Can you work these out from the model? Positions are in its coordinate system, mm. A direction names the side the tool comes from. Give positions to 0.01 mm unless a question says otherwise; leave off trailing zeros. Write each loop counter-clockwise with the first axis right and the second up, starting at its lowest first coordinate (ties: lowest second). Pieces come first, ordered by that corner, then holes.
```python
from build123d import *

# Parameters (mm, degrees)
F1_DEPTH = 5.08
F2_R     = 2.6137383635
F2_R_2   = 1.27
F3_DEPTH = 1.016
F5_DEPTH = 0.4572
F6_R     = 1.5849178859
F6_R_2   = 1.5875
F7_DEPTH = 1.27
F9_DEPTH = 1.27


with BuildPart() as f1:
    # F0 (on Top) → F1 (new body)
    with BuildSketch(Plane.XY):
        with BuildLine():
            Line((-3.2727682094, 26.3807782884), (-6.4659603156, 19.0687214415))
            Line((-6.4659603156, 19.0687214415), (-30.863808468, 9.4360690564))
            ThreePointArc((-30.863808468, 9.4360690564), (-32.5086762666, 4.4664752799), (-27.325283736, 3.7351106293))
            Line((-27.325283736, 3.7351106293), (-6.8804663606, 11.2053323537))
            Line((-6.8804663606, 11.2053323537), (-6.8804663606, -7.0770513266))
            Line((-6.8804663606, -7.0770513266), (-21.0345704108, -28.5047926009))
            ThreePointArc((-21.0345704108, -28.5047926009), (-17.4572264743, -34.3414996844), (-11.008746922, -32.0433154702))
            Line((-11.008746922, -32.0433154702), (0, -13.9575190842))
            Line((0, -13.9575190842), (11.008746922, -32.0433154702))
            ThreePointArc((11.008746922, -32.0433154702), (17.4572264743, -34.3414996844), (21.0345704108, -28.5047926009))
            Line((21.0345704108, -28.5047926009), (6.8804663606, -7.0770513266))
            Line((6.8804663606, -7.0770513266), (6.8804663606, 11.2053323537))
            Line((6.8804663606, 11.2053323537), (27.325283736, 3.7351106293))
            ThreePointArc((27.325283736, 3.7351106293), (32.5086762666, 4.4664752799), (30.863808468, 9.4360690564))
            Line((30.863808468, 9.4360690564), (6.4659603156, 19.0687214415))
            Line((6.4659603156, 19.0687214415), (3.2727682094, 26.3807782884))
            ThreePointArc((3.2727682094, 26.3807782884), (0, 44.2043436195), (-3.2727682094, 26.3807782884))
        make_face()
    extrude(amount=F1_DEPTH)

    # F2 (on face) → F3 (join)
    with BuildSketch(Plane.XY.offset(5.08)):
        with Locations((-4.7121047974, 37.2473150492)):
            Circle(F2_R)
        with Locations((-4.7121047974, 37.2473150492)):
            Circle(F2_R_2, mode=Mode.SUBTRACT)
        with Locations((4.7121047974, 37.2473150492)):
            Circle(F2_R)
        with Locations((4.7121047974, 37.2473150492)):
            Circle(F2_R_2, mode=Mode.SUBTRACT)
        with BuildLine():
            Line((-3.2727682094, 30.2372745808), (-4.7121047974, 32.4515290558))
            ThreePointArc((-4.7121047974, 32.4515290558), (0.2937612268, 27.1153177061), (5.2996272509, 32.4515290558))
            Line((5.2996272509, 32.4515290558), (3.2727682094, 30.2372745808))
            Line((3.2727682094, 30.2372745808), (2.0341726185, 32.4515290558))
            Line((2.0341726185, 32.4515290558), (0, 30.2372745808))
            Line((0, 30.2372745808), (-1.5411652881, 32.4515290558))
            Line((-1.5411652881, 32.4515290558), (-3.2727682094, 30.2372745808))
        make_face()
        Polygon((-1.5411652881, 32.4515290558), (-4.7121047974, 32.4515290558), (-3.2727682094, 30.2372745808), align=None)
        Polygon((3.2727682094, 30.2372745808), (5.2996272509, 32.4515290558), (2.0341726185, 32.4515290558), align=None)
        Polygon((2.0341726185, 32.4515290558), (-1.5411652881, 32.4515290558), (0, 30.2372745808), align=None)
    extrude(amount=F3_DEPTH)

    # F4 (on face) → F5 (join)
    with BuildSketch(Plane.XY.offset(6.096)):
        with BuildLine():
            Line((-3.2727682094, 30.2372745808), (-4.7121047974, 32.4515290558))
            ThreePointArc((-4.7121047974, 32.4515290558), (-4.7203324358, 32.2729584869), (-4.7221920847, 32.0942081475))
            Line((-4.7221920847, 32.0942081475), (-3.4431374496, 30.126529098))
            Line((-3.4431374496, 30.126529098), (-3.2880254188, 29.8879070055))
            Line((-3.2880254188, 29.8879070055), (-3.1127018776, 30.1120986668))
            Line((-3.1127018776, 30.1120986668), (-1.5506819831, 32.1095020547))
            Line((-1.5506819831, 32.1095020547), (-0.1667791776, 30.121192946))
            Line((-0.1667791776, 30.121192946), (-0.0219153894, 29.9130612851))
            Line((-0.0219153894, 29.9130612851), (0.1496401921, 30.0998043917))
            Line((0.1496401921, 30.0998043917), (1.9938853204, 32.1073174174))
            Line((1.9938853204, 32.1073174174), (3.0954276532, 30.138074948))
            Line((3.0954276532, 30.138074948), (3.2517947624, 29.9134160007))
            Line((3.2517947624, 29.9134160007), (3.4226548069, 30.1000730943))
            Line((3.4226548069, 30.1000730943), (5.3097613024, 32.1616540513))
            ThreePointArc((5.3097613024, 32.1616540513), (5.306789943, 32.3066648182), (5.2996272509, 32.4515290558))
            Line((5.2996272509, 32.4515290558), (3.2727682094, 30.2372745808))
            Line((3.2727682094, 30.2372745808), (2.13859977, 32.2648431922))
            Line((2.13859977, 32.2648431922), (2.0341726185, 32.4515290558))
            Line((2.0341726185, 32.4515290558), (1.8894581688, 32.2940032811))
            Line((1.8894581688, 32.2940032811), (0, 30.2372745808))
            Line((0, 30.2372745808), (-1.4196918326, 32.2770032315))
            Line((-1.4196918326, 32.2770032315), (-1.5411652881, 32.4515290558))
            Line((-1.5411652881, 32.4515290558), (-1.6721554386, 32.2840278791))
            Line((-1.6721554386, 32.2840278791), (-3.2727682094, 30.2372745808))
        make_face()
    extrude(amount=F5_DEPTH)

    # F6 (on face) → F7 (join)
    with BuildSketch(Plane.XY.offset(5.08)):
        with Locations((0, 16.6316951297)):
            Circle(F6_R)
        with Locations((0, 10.2816951297)):
            Circle(F6_R_2)
        with Locations((0, 3.9316951297)):
            Circle(F6_R_2)
    extrude(amount=F7_DEPTH)

    # F8 (on face) → F9 (join)
    with BuildSketch(Plane.XY.offset(5.08)):
        with BuildLine():
            add(Edge.make_bspline(
                [(-7.0363054983, -4.8071318306), (-6.9812030221, -5.5234641768), (-6.9261005459, -6.239796523), (-6.8709980696, -6.9561288692)],
                knots=[0, 0, 0, 0, 2.1553456377, 2.1553456377, 2.1553456377, 2.1553456377], degree=3))
            add(Edge.make_bspline(
                [(-6.8709980696, -6.9561288692), (-5.6130342711, -8.3738225884), (-3.1848892901, -11.1102812153), (-0.243495057, -7.0612015798), (4.5821148023, -4.8991787577), (6.1734744422, -6.3428325856), (6.8495194428, -6.9561288692)],
                knots=[0, 0, 0, 0, 0.2686113424, 0.5184785791, 0.7954389812, 1, 1, 1, 1], degree=3))
            add(Edge.make_bspline(
                [(-7.0363054983, -4.8071318306), (-5.7248109737, -6.1236047459), (-3.2262965612, -8.6316034379), (-0.1133011688, -5.1968632917), (4.3194928458, -2.8270018136), (7.3601699927, -4.4068743135), (7.0165421861, -6.1223228754), (6.8495194428, -6.9561288692)],
                knots=[0, 0, 0, 0, 0.2276234559, 0.4336430496, 0.668963168, 0.8390971896, 1, 1, 1, 1], degree=3))
        make_face()
    extrude(amount=F9_DEPTH)


solid = f1.part
```
1) For pin 1 Ø2.5 at (x, y) = (5, 37.5) entering from +Z; pin 2 Ø3 at (y, z) = (29.5, 4) entering from +X; pin 3 Ø1 at (x, y) = (-5.5, 5.5) entering from +Z; pin 4 Ø5 at (x, y) = (-11, 7.5) entering from -Z, each with a flat end and sliding along its axis, tell me the tip position at first contact or that it passes through.
Values follow:
pin 1: stops at z = 6.1
pin 2: stops at x = 8.3
pin 3: stops at z = 5.08
pin 4: stops at z = 0
2) For faces 1 (the face through (0.2, 29.7, 6.096)), 2 (the face through (-13.86, -17.64, 2.5)), 3 (the face through (4, 32, 6.096)), which set-ups out of +Z, -Z, +X, -X, +Y, -Y let a thin tool reach every point of the face, with its end or its side?
Values follow:
face 1: +Z
face 2: +Z, -Z, -X
face 3: +Z, +Y
3) Suppose I cut it at B-B on x = -13. Write out the boundary of the cut face in (y, z), plus the area to 3 significant figures.
Values follow:
outline: (-33.96, 0) - (-16.34, 0) - (-16.34, 5.08) - (-33.96, 5.08) - close; (8.97, 0) - (16.49, 0) - (16.49, 5.08) - (8.97, 5.08) - close
area: 128 mm2
4) Suppose I cut it at C-C on y = -27.5. Write out the boundary of the cut face in (x, z).
Values follow:
outline: (-20.37, 0) - (-8.24, 0) - (-8.24, 5.08) - (-20.37, 5.08) - close; (8.24, 0) - (20.37, 0) - (20.37, 5.08) - (8.24, 5.08) - close
5) Please list where these lines run through material, in increasing order: L1, parallel to Y at x = -8.5, z = 0.5; L2, parallel to Y at x = -8, z = 3.5; L3, parallel to Y at x = 3.5, z = 5.
Values follow:
L1: y = -27.92 to -9.53, 10.61 to 18.27, 31.44 to 38.54
L2: y = -27.1 to -8.77, 10.8 to 18.46, 30.42 to 39.56
L3: y = -19.71 to 25.86, 26.47 to 43.51
6) Suppose I cut it at A-A on z = 1. Write out the boundary of the cut face in (x, y) (1 decimal), plus the area to 3 significant figures.
Values follow:
outline: (-30.9, 9.4) arc R3.4 ccw (long way) to (-27.3, 3.7) - (-6.9, 11.2) - (-6.9, -7.1) - (-21, -28.5) arc R5.4 ccw to (-11, -32) - (0, -14) - (11, -32) arc R5.4 ccw to (21, -28.5) - (6.9, -7.1) - (6.9, 11.2) - (27.3, 3.7) arc R3.4 ccw (long way) to (30.9, 9.4) - (6.5, 19.1) - (3.3, 26.4) arc R9.2 ccw (long way) to (-3.3, 26.4) - (-6.5, 19.1) - close
area: 1,650 mm2
7) If we mould it in two halves opening along X, with no side actions, what happens to faces 4 (the face through (6, 38, 6.096)), 5 (the face through (4.3, 31.36, 6.32)), 6 (the face through (-0.206, 18.203, 5.706)), 7 (the face through (-6.64, 39.01, 5.58))? For each: +X half, -X half, draft (parallel to the pull), parting line (faces both ways), or undercut.
Values follow:
face 4: draft
face 5: undercut
face 6: parting line
face 7: undercut
8) Suppose I cut it at D-D on x = 22. Write out the boundary of the cut face in (y, z), plus the area to 3 significant figures.
Values follow:
outline: (5.68, 0) - (12.94, 0) - (12.94, 5.08) - (5.68, 5.08) - close
area: 36.9 mm2
